from build123d import *

# Parameters (mm, degrees)
BOSS_EXTRUDE1_DEPTH    = 1.016
CUT_EXTRUDE1_DEPTH     = 78.144111272
FILLET1_R              = 0.635
FILLET2_R              = 1.27
FILLET3_R              = 0.635
SKETCH3_R              = 1.397
CUT_EXTRUDE2_DEPTH     = 78.144111272
CUT_EXTRUDE3_DEPTH     = 0.360211591
CUT_EXTRUDE3_TAPER     = 20
FILLET4_R              = 0.254
FILLET5_R              = 3.175
SKETCH5_R              = 0.889
CUT_EXTRUDE4_DEPTH     = 78.144111382
CUT_EXTRUDE5_OUTLINE_W = 0.508
CUT_EXTRUDE5_OUTLINE_H = 11.08
CUT_EXTRUDE5_DEPTH     = 34.163


# Read off the part's stored shape, not the designer's step: Cut-Extrude3, Cut-Extrude5
with BuildPart() as part:
    # Sketch1 → Boss-Extrude1 (new body)
    with BuildSketch(Plane(origin=(0, 0, 0), x_dir=(1, 0, 0), z_dir=(0, 1, 0))):
        with BuildLine():
            Line((0, 0), (19.05, 0))
            Line((19.05, 0), (19.05, 2.032))
            Line((19.05, 2.032), (27.94, 2.032))
            ThreePointArc((27.94, 2.032), (31.279316908, 2.659542662), (34.163, 4.456545455))
            ThreePointArc((34.163, 4.456545455), (37.719, 5.842), (41.275, 4.456545455))
            ThreePointArc((41.275, 4.456545455), (44.158683092, 2.659542662), (47.498, 2.032))
            Line((47.498, 2.032), (67.818, 2.032))
            Line((67.818, 2.032), (67.818, -0.508))
            Line((67.818, -0.508), (75.687113577, -0.508))
            ThreePointArc((75.687113577, -0.508), (76.708, -4.318), (75.687113577, -8.128))
            Line((75.687113577, -8.128), (62.738, -8.128))
            Line((62.738, -8.128), (62.738, -4.318))
            Line((62.738, -4.318), (54.61, -4.318))
            ThreePointArc((54.61, -4.318), (52.813948776, -3.574051224), (52.07, -1.778))
            Line((52.07, -1.778), (52.07, -0.508))
            Line((52.07, -0.508), (31.75, -0.508))
            Line((31.75, -0.508), (31.75, -5.08))
            Line((31.75, -5.08), (10.472688289, -5.08))
            ThreePointArc((10.472688289, -5.08), (4.652817156, -3.742971704), (0, 0))
        make_face()
    extrude(amount=BOSS_EXTRUDE1_DEPTH)

    # Sketch2 → Cut-Extrude1 (cut, through all)
    with BuildSketch(Plane(origin=(0, 1.016, 0), x_dir=(1, 0, 0), z_dir=(0, 1, 0))):
        with BuildLine():
            Line((52.959, -1.778), (52.07, -1.778))
            Line((52.07, -1.778), (52.07, -0.508))
            Line((52.07, -0.508), (52.959, -0.508))
            ThreePointArc((52.959, -0.508), (53.594, -1.143), (52.959, -1.778))
        make_face()
    extrude(amount=-CUT_EXTRUDE1_DEPTH, mode=Mode.SUBTRACT)

    # Fillet1
    fillet1_edges = [part.edges().sort_by_distance(p)[0] for p in [
        (52.07, 0.508, 1.778),
    ]]
    fillet(fillet1_edges, radius=FILLET1_R)

    # Fillet2
    fillet2_edges = [part.edges().sort_by_distance(p)[0] for p in [
        (67.818, 0.508, 0.508),
        (67.818, 0.508, -2.032),
        (62.738, 0.508, 8.128),
        (62.738, 0.508, 4.318),
        (31.75, 0.508, 5.08),
    ]]
    fillet(fillet2_edges, radius=FILLET2_R - 0.0001)  # a hair under: the kernel refuses the full size

    # Fillet3
    fillet3_edges = [part.edges().sort_by_distance(p)[0] for p in [
        (19.05, 0.508, 0),
        (19.05, 0.508, -2.032),
        (75.687113577, 0.508, 0.508),
        (75.687113577, 0.508, 8.128),
    ]]
    fillet(fillet3_edges, radius=FILLET3_R)

    # Sketch3 → Cut-Extrude2 (cut, through all)
    with BuildSketch(Plane(origin=(0, 1.016, 0), x_dir=(1, 0, 0), z_dir=(0, 1, 0))):
        with Locations(Location((71.755, -3.937, 0), (0, 0, 270))):
            Circle(SKETCH3_R)
    extrude(amount=-CUT_EXTRUDE2_DEPTH, mode=Mode.SUBTRACT)

    # Cut-Extrude3 outline → Cut-Extrude3 (cut)
    with BuildSketch(Plane(origin=(0, -0.296094575, -0.079338302), x_dir=(-1, 0, 0), z_dir=(0, 0.9659258262890681, 0.25881904510252135))):
        with BuildLine():
            ThreePointArc((-34.967158874, -4.659244146), (-37.719, -3.594110297), (-40.470841126, -4.659244146))
            Line((-40.470841126, -4.659244146), (-34.967158874, -4.659244146))
        make_face()
    extrude(amount=CUT_EXTRUDE3_DEPTH, taper=CUT_EXTRUDE3_TAPER, mode=Mode.SUBTRACT)

    # Fillet4
    fillet4_edges = [part.edges().sort_by_distance(p)[0] for p in [
        (37.719, 0.63412962, -3.55098226),
    ]]
    fillet(fillet4_edges, radius=FILLET4_R - 0.0001)  # a hair under: the kernel refuses the full size

    # Fillet5
    fillet5_edges = [part.edges().sort_by_distance(p)[0] for p in [
        (31.75, 0.508, 0.508),
    ]]
    fillet(fillet5_edges, radius=FILLET5_R)

    # Sketch5 → Cut-Extrude4 (cut, through all)
    with BuildSketch(Plane(origin=(0, 1.016, 0), x_dir=(1, 0, 0), z_dir=(0, 1, 0))):
        with Locations(Location((29.21, -1.397, 0), (0, 0, 270))):
            Circle(SKETCH5_R)
    extrude(amount=-CUT_EXTRUDE4_DEPTH, mode=Mode.SUBTRACT)

    # Cut-Extrude5 outline → Cut-Extrude5 (cut)
    with BuildSketch(Plane.YZ):
        with Locations((0.254, -0.46)):
            Rectangle(CUT_EXTRUDE5_OUTLINE_W, CUT_EXTRUDE5_OUTLINE_H)
    extrude(amount=CUT_EXTRUDE5_DEPTH, mode=Mode.SUBTRACT)


solid = part.part
Read the model definition and answer for the solid it produces. Units are mm, in the model's axes. A direction names the side the tool comes from. Round coordinates to 2 decimals unless told otherwise and drop trailing zeros. Write each loop counter-clockwise with the first axis right and the second up, starting at its lowest first coordinate (ties: lowest second). Pieces come first, ordered by that corner, then holes.
1. Determine the mould class of faces 4 (the face through (62.356, 0.515, 4.68)), 5 (the face through (73.14, 0.52, 3.76)), 6 (the face through (31.23, 0.76, -2.64)) for opening direction Z: pulls with the +Z half, pulls with the -Z half, needs draft (parallel to the pull), parting line crosses it, or undercut.
2. Straight lines are drawn through the part: L1, parallel to Z at x = 11.5, y = 0.65; L2, parallel to Y at x = 30.5, z = -1; L3, parallel to Z at x = 51, y = 0.15. For each, find the intervals that lie inside material, in ascending order.
3. Given pin 1 Ø0.6 at (y, z) = (0.5, -1) entering from -X; pin 2 Ø6 at (x, z) = (28.5, 3.5) entering from -Y; pin 3 Ø0.5 at (x, y) = (59.5, 0.5) entering from +Z; pin 4 Ø1.1 at (x, z) = (29.21, 1.397) entering from +Y, each flat-ended and moving along its own axis, determine where each tip first touches the part or whether it passes through.
4. The part is cut by section C-C, the plane x = 51.5. Determine the outline of the cut face in (y, z), then the cut area to 3 significant figures.
5. The part is cut by section B-B, the plane x = 29.21. Determine the outline of the cut face in (y, z), then the cut area to 3 significant figures.
6. Which of the six approach directions +Z, -Z, +X, -X, +Y, -Y give full straight-line access (tool end or side, diameter ignored) to faces 1 (the face through (32.705, 0.741, 1.413)), 2 (the face through (44.11, 0.5, -2.68)), 3 (the face through (21, 0.508, 1))?
Values:
1. face 4: pulls with the +Z half
1. face 5: undercut
1. face 6: pulls with the -Z half
2. L1: z = 0 to 5.08
2. L2: y = 0.51 to 1.02
2. L3: z = -2.03 to 0.51
3. pin 1: stops at x = 19.05
3. pin 2: stops at y = 0.51
3. pin 3: stops at z = 4.32
3. pin 4: passes through
4. outline: (0, -2.03) - (1.02, -2.03) - (1.02, 0.51) - (0, 0.51) - close
4. area: 2.58 mm2
5. outline: (0.51, -2.12) - (1.02, -2.12) - (1.02, 0.51) - (0.51, 0.51) - close; (0.51, 2.29) - (1.02, 2.29) - (1.02, 5.08) - (0.51, 5.08) - close
5. area: 2.75 mm2
6. face 1: +Z, +Y, -Y
6. face 2: -Z, +X, +Y, -Y
6. face 3: +Z, -Z, -X, -Y
